```python
from build123d import *

# Parameters (mm, degrees)
F0_W     = 120
F0_H     = 90
F1_DEPTH = 5
F3_DEPTH = 5
F4_R     = 30
F5_DEPTH = 5
F6_R     = 3
F7_DEPTH = 25


with BuildPart() as f1:
    # F0 (on Top) → F1 (new body)
    with BuildSketch(Plane.XY):
        with Locations((-60, 45)):
            Rectangle(F0_W, F0_H)
    extrude(amount=F1_DEPTH)

    # F2 (on face) → F3 (join)
    with BuildSketch(Plane.XY.offset(5)):
        with BuildLine():
            Line((-10, 27), (-5, 27))
            Line((-5, 27), (-5, 70))
            ThreePointArc((-5, 70), (-9.393398, 80.606602), (-20, 85))
            Line((-20, 85), (-105, 85))
            Line((-105, 85), (-115, 63))
            Line((-115, 63), (-115, 27))
            Line((-115, 27), (-110, 27))
            ThreePointArc((-110, 27), (-99.393398, 22.606602), (-95, 12))
            Line((-95, 12), (-95, 5))
            Line((-95, 5), (-25, 5))
            Line((-25, 5), (-25, 12))
            ThreePointArc((-25, 12), (-20.606602, 22.606602), (-10, 27))
        make_face()
    extrude(amount=F3_DEPTH)

    # F4 (on face) → F5 (cut)
    with BuildSketch(Plane.XY.offset(10)):
        with Locations((-60, 45)):
            Circle(F4_R)
    extrude(amount=-F5_DEPTH, mode=Mode.SUBTRACT)

    # F6 (on face) → F7 (cut)
    with BuildSketch(Plane.XY.offset(10)):
        with Locations((-80, 45)):
            Circle(F6_R)
        with Locations((-60, 25)):
            Circle(F6_R)
        with Locations((-60, 65)):
            Circle(F6_R)
        with Locations((-40, 45)):
            Circle(F6_R)
        with Locations((-74.14, 59.144271)):
            Circle(F6_R)
        with Locations((-45.86, 59.144271)):
            Circle(F6_R)
        with Locations((-74.14, 30.855729)):
            Circle(F6_R)
        with Locations((-45.86, 30.855729)):
            Circle(F6_R)
    extrude(amount=-F7_DEPTH, mode=Mode.SUBTRACT)


solid = f1.part
```
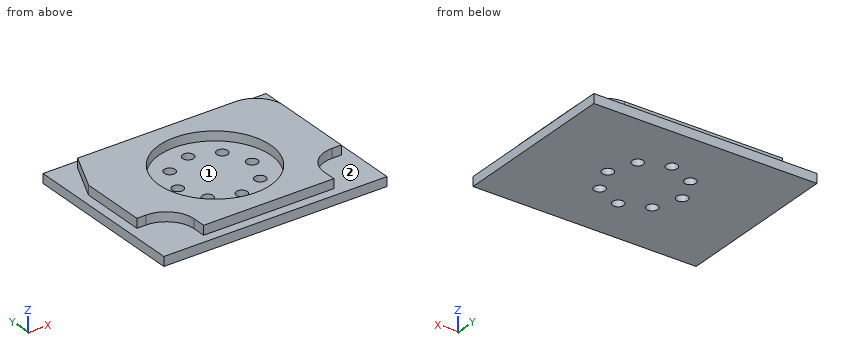
Source: CAD feature listing. Evaluate the final solid. Frame: model axes, mm. Face numbers are marked on the shaded views. Give positions to 0.01 mm unless a question says otherwise; leave off trailing zeros. Order: outer loops, then holes, each group sorted by start corner. A loop starts at its lowest first (then second) coordinate and runs counter-clockwise, first axis right, second up.
(1) Section query D-D (x = -40). Return the cut outline in (y, z).
(2) Section query A-A (y = 45). Return the cut outline in (x, z), plus the area to 3 significant figures.
(3) Section query C-C (z = 7.75). Return the cut outline in (x, y), plus the area to 3 significant figures.
(4) Material intervals for line 1 along Y through (x, z) = (-60, 3.8); line 2 along Y through (x, z) = (-45.86, 3.35); line 3 along Z through (x, y) = (-73, 70.5), sorted ascending.
(5) Contact query for flat-ended pins moving along their axis: P1, Ø5, axis at y = 15, z = 7, coming from the +X side; P2, Ø6, axis at x = -40.5, y = 52, coming from the +Z side; P3, Ø2.5, axis at y = 46.5, z = 8.5, coming from the +X side; P4, Ø1.5, axis at x = -57, z = 6.5, coming from the +Y side. Output: stop coordinate, or through.
(6) Pull-direction query (X, two-part tool) for the marked faces 1 and 2; classes: +X half, -X half, draft (parallel to the pull), parting line (faces both ways), or undercut.
(7) Section query B-B (x = -60). Return the cut outline in (y, z).
Outcome:
1. outline: (0, 0) - (42, 0) - (42, 5) - (22.64, 5) - (22.64, 10) - (5, 10) - (5, 5) - (0, 5) - close; (48, 0) - (90, 0) - (90, 5) - (85, 5) - (85, 10) - (67.36, 10) - (67.36, 5) - (48, 5) - close
2. outline: (-120, 0) - (-83, 0) - (-83, 5) - (-90, 5) - (-90, 10) - (-115, 10) - (-115, 5) - (-120, 5) - close; (-77, 0) - (-43, 0) - (-43, 5) - (-77, 5) - close; (-37, 0) - (0, 0) - (0, 5) - (-5, 5) - (-5, 10) - (-30, 10) - (-30, 5) - (-37, 5) - close
2. area: 790 mm2
3. outline: (-115, 27) - (-110, 27) arc R15 cw to (-95, 12) - (-95, 5) - (-25, 5) - (-25, 12) arc R15 cw to (-10, 27) - (-5, 27) - (-5, 70) arc R15 ccw to (-20, 85) - (-105, 85) - (-115, 63) - close; hole circle Ø60 at (-60, 45)
3. area: 5,030 mm2
4. line 1: y = 0 to 22, 28 to 62, 68 to 90
4. line 2: y = 0 to 27.86, 33.86 to 56.14, 62.14 to 90
4. line 3: z = 0 to 5
5. P1: stops at x = 0
5. P2: stops at z = 5
5. P3: stops at x = -5
5. P4: stops at y = 85
6. face 1: undercut
6. face 2: draft
7. outline: (0, 0) - (22, 0) - (22, 5) - (15, 5) - (15, 10) - (5, 10) - (5, 5) - (0, 5) - close; (28, 0) - (62, 0) - (62, 5) - (28, 5) - close; (68, 0) - (90, 0) - (90, 5) - (85, 5) - (85, 10) - (75, 10) - (75, 5) - (68, 5) - close
